Build history of the part. All positions in model axes, mm. Face numbers are marked on the shaded views. A direction names the side the tool comes from. Round coordinates to 2 decimals unless told otherwise and drop trailing zeros. Loops run counter-clockwise (first coordinate to the right, second up) from the corner with the lowest first, then second, coordinate; pieces in that order, holes last. Notation, with made-up numbers: (21, 19) - (45, 19) arc R20 cw to (45, 40) - close; hole circle Ø6 at (88.5, -20.5). An arc over 180 degrees is marked (long way). Answer as CSV lines item,"result". Start each with the question number.
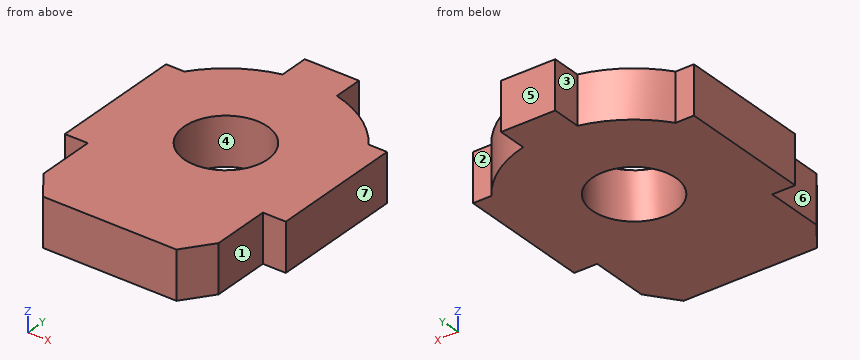
Autodesk Inventor part; units mm, degrees
ref_plane "YZ Plane" through (0, 0, 0) normal (1, 0, 0) x (0, 1, 0)
ref_plane "XZ Plane" through (0, 0, 0) normal (0, 1, 0) x (-1, 0, 0)
ref_plane "XY Plane" through (0, 0, 0) normal (0, 0, 1) x (1, 0, 0)
sketch "Sketch1" plane through (0, 0, 0) normal (0, 0, 1) x (1, 0, 0)
  circle A0 centre (0, 0) radius 2
  line L0 (-5.3, 3.2) -> (-5.3, -3.2)
  line L1 (-5.3, -3.2) -> (-4.2, -3.2)
  line L2 (-4.2, -3.2) -> (-4.2, -6)
  line L3 (-4.2, -6) -> (-3.2, -7.35)
  line L4 (-3.2, -7.35) -> (0, -7.35)
  line L5 (-1.3, 6.7) -> (-1.3, 5.3)
  line L6 (-1.3, 6.7) -> (0, 6.7)
  line L7 (0, 5.3) -> (0, -7.35) construction
  arc A1 (-1.3, 5.3) -> (-4.4204, 3.2) centre (0, 0) ccw
  line L8 (-5.3, 3.2) -> (-4.4204, 3.2)
  line L9 (0, 0) -> (-5.3, 0) construction
  line L10 (5.3, 3.2) -> (5.3, -3.2)
  line L11 (5.3, -3.2) -> (4.2, -3.2)
  line L12 (4.2, -3.2) -> (4.2, -6)
  line L13 (4.2, -6) -> (3.2, -7.35)
  line L14 (3.2, -7.35) -> (0, -7.35)
  line L15 (1.3, 6.7) -> (1.3, 5.3)
  line L16 (1.3, 6.7) -> (0, 6.7)
  arc A2 (4.4204, 3.2) -> (1.3, 5.3) centre (0, 0) ccw
  line L17 (5.3, 3.2) -> (4.4204, 3.2)
  line L18 (0, 0) -> (5.3, 0) construction
  dimension "d0" = 4
  dimension "d1" = 1.3
  dimension "d2" = 5.3
  dimension "d3" = 6.7
  dimension "d4" = 4.2
  dimension "d5" = 5.3
  dimension "d7" = 3.2
  dimension "d9" = 7.35
  dimension "d10" = 3.2
  dimension "d11" = 2.8
extrude "Extrusion1" add sketch "Sketch1" along normal blind 2.3
properties part number "encoder_coarse"
Q1. Band-saw the part on A-A, the plane z = 0.95. List the corners of the cut face in (x, y), then the cut area to 3 significant figures.
Q2. Tool access for the marked faces 1, 2 and 3: list every direction of +Z, -Z, +X, -X, +Y, -Y with a clear straight run to the whole face (end or side of a thin tool).
Q3. Band-saw the part on C-C, the plane y = 0. List the corners of the cut face in (x, z).
Q4. Two-plate mould, pull along X, no slides. Class the marked faces 4, 5, 6 and 7: released by +X, released by -X, zero draft, split by the parting line, or undercut.
Q5. Pin check, flat tips, straight feed: pin 1 Ø1.2 at (x, z) = (4.5, 1) entering from -Y (3 decimals); pin 2 Ø3 at (x, y) = (0, 0) entering from -Z; pin 3 Ø1.2 at (y, z) = (-5, 1.5) entering from -X; pin 4 Ø1.2 at (y, z) = (-4.5, 1) entering from +X. Stop position of each tip, or through.
Q6. Band-saw the part on D-D, the plane y = -5. List the corners of the cut face in (x, z), then the cut area to 3 significant figures.
Q7. Band-saw the part on B-B, the plane x = 0. List the corners of the cut face in (y, z), then the cut area to 3 significant figures.
Q8. Wall check: probe 1 along Y at (x, z) = (0, 1.1); probe 2 along X at (y, z) = (-1.75, 1.95); probe 3 along X at (y, z) = (-1.5, 1.7). Give the ranges that are in metal, low to high. Write a range as [from, to].
Reported:
1,outline,"(-5.3, -3.2) - (-4.2, -3.2) - (-4.2, -6) - (-3.2, -7.35) - (3.2, -7.35) - (4.2, -6) - (4.2, -3.2) - (5.3, -3.2) - (5.3, 3.2) - (4.42, 3.2) arc R5.46 ccw to (1.3, 5.3) - (1.3, 6.7) - (-1.3, 6.7) - (-1.3, 5.3) arc R5.46 ccw to (-4.42, 3.2) - (-5.3, 3.2) - close; hole circle Ø4 at (0, 0)"
1,area,"106 mm2"
2,face 1,"+Z, -Z, +X, -Y"
2,face 2,"+Z, -Z, +X, +Y"
2,face 3,"+Z, -Z, -X, +Y"
3,outline,"(-5.3, 0) - (-2, 0) - (-2, 2.3) - (-5.3, 2.3) - close; (2, 0) - (5.3, 0) - (5.3, 2.3) - (2, 2.3) - close"
4,face 4,"undercut"
4,face 5,"zero draft"
4,face 6,"released by -X"
4,face 7,"released by +X"
5,pin 1,"stops at y = -6.405"
5,pin 2,"passes through"
5,pin 3,"stops at x = -4.2"
5,pin 4,"stops at x = 4.2"
6,outline,"(-4.2, 0) - (4.2, 0) - (4.2, 2.3) - (-4.2, 2.3) - close"
6,area,"19.3 mm2"
7,outline,"(-7.35, 0) - (-2, 0) - (-2, 2.3) - (-7.35, 2.3) - close; (2, 0) - (6.7, 0) - (6.7, 2.3) - (2, 2.3) - close"
7,area,"23.1 mm2"
8,probe 1,"y = [-7.35, -2], [2, 6.7]"
8,probe 2,"x = [-5.3, -0.97], [0.97, 5.3]"
8,probe 3,"x = [-5.3, -1.32], [1.32, 5.3]"
